Autodesk Inventor part; units mm, degrees
ref_plane "Work Plane1" through (28, 0, 0) normal (1, 0, 0) x (0, 1, 0)
ref_plane "XZ Plane" through (0, 0, 0) normal (0, 1, 0) x (-1, 0, 0)
ref_plane "XY Plane" through (0, 0, 0) normal (0, 0, 1) x (1, 0, 0)
sketch "Sketch1" plane through (0, 0, 0) normal (1, 0, 0) x (0, 1, 0)
  line L0 (-21.15, 21.15) -> (21.15, 21.15)
  line L1 (21.15, 21.15) -> (21.15, -21.15)
  line L2 (21.15, -21.15) -> (-21.15, -21.15)
  line L3 (-21.15, -21.15) -> (-21.15, 21.15)
  point P0 (0, 0)
  point P1 (0, 21.15)
  point P2 (21.15, 0)
  dimension "d0" = 42.3
  dimension "d1" = 42.3
extrude "Extrusion1" add sketch "Sketch1" along normal mid plane 56
ref_plane "Work Plane1" through (28, 0, 0) normal (1, 0, 0) x (0, 1, 0)
sketch "Sketch2" plane through (28, 0, 0) normal (1, 0, 0) x (0, 1, 0)
  circle A0 centre (0, 0) radius 11
  circle A1 centre (0, 0) radius 2.5
  circle A2 centre (15.5, 15.5) radius 2.55
  line L0 (21.15, -21.15) -> (21.15, 21.15) construction
  line L1 (21.15, 0) -> (0, 0) construction
  line L2 (0, 0) -> (0, 21.15) construction
  line L3 (21.15, 21.15) -> (-21.15, 21.15) construction
  circle A3 centre (15.5, -15.5) radius 2.55
  circle A4 centre (-15.5, 15.5) radius 2.55
  circle A5 centre (-15.5, -15.5) radius 2.55
  line L4 (1, 2.2913) -> (1, -2.2913)
  dimension "d5" = 22
  dimension "d6" = 5
  dimension "d15" = 5.1
  dimension "d16" = 31
  dimension "d17" = 31
  dimension "d20" = 1
extrude "Extrusion2" add sketch "Sketch2" along normal blind 2 contours A0
fillet "Fillet1" radius 2 1 edges at (0, 21.15, 21.15)
pattern_circular "Circular Pattern1" count 4 over 360 about axis through (28, 0, 0) along (1, 0, 0) of "Fillet1"
extrude "Extrusion4" cut sketch "Sketch2" against normal through all contours A2 | A3 | A4 | A5
sketch "Sketch3" plane through (0, 0, 0) normal (1, 0, 0) x (0, 1, 0)
  circle A0 centre (-15.5, 15.5) radius 2.55 construction
  circle A1 centre (15.5, 15.5) radius 2.55 construction
  circle A2 centre (-15.5, -15.5) radius 2.55 construction
  circle A3 centre (15.5, -15.5) radius 2.55 construction
  arc A4 (19.15, -21.15) -> (21.15, -19.15) centre (19.15, -19.15) ccw construction
  line L0 (21.15, -19.15) -> (21.15, 19.15) construction
  arc A5 (21.15, 19.15) -> (19.15, 21.15) centre (19.15, 19.15) ccw construction
  line L1 (19.15, 21.15) -> (-19.15, 21.15) construction
  arc A6 (-19.15, 21.15) -> (-21.15, 19.15) centre (-19.15, 19.15) ccw construction
  line L2 (-21.15, 19.15) -> (-21.15, -19.15) construction
  arc A7 (-21.15, -19.15) -> (-19.15, -21.15) centre (-19.15, -19.15) ccw construction
  line L3 (-19.15, -21.15) -> (19.15, -21.15) construction
  circle A8 centre (0, 0) radius 11 construction
  circle A9 centre (15.5, 15.5) radius 5.65 construction
  line L4 (-19.15, 21.15) -> (19.15, 21.15) construction
  line L5 (0, 21.15) -> (0, 0) construction
  line L6 (0, 0) -> (21.15, 0) construction
  line L7 (9.85, 15.5) -> (9.85, 21.15)
  line L8 (9.85, 21.15) -> (21.15, 21.15)
  line L9 (21.15, 21.15) -> (21.15, 9.85)
  line L10 (15.5, 9.85) -> (21.15, 9.85)
  arc A10 (9.85, 15.5) -> (15.5, 9.85) centre (15.5, 15.5) ccw
  circle A11 centre (15.5, -15.5) radius 2.55 construction
  arc A12 (19.15, -21.15) -> (21.15, -19.15) centre (19.15, -19.15) ccw construction
  circle A13 centre (0, 0) radius 11 construction
  circle A14 centre (15.5, -15.5) radius 5.65 construction
  line L11 (-19.15, -21.15) -> (19.15, -21.15) construction
  line L12 (9.85, -15.5) -> (9.85, -21.15)
  line L13 (9.85, -21.15) -> (21.15, -21.15)
  line L14 (21.15, -21.15) -> (21.15, -9.85)
  line L15 (15.5, -9.85) -> (21.15, -9.85)
  arc A15 (15.5, -9.85) -> (9.85, -15.5) centre (15.5, -15.5) ccw
  circle A16 centre (-15.5, 15.5) radius 2.55 construction
  circle A17 centre (-15.5, -15.5) radius 2.55 construction
  arc A18 (-21.15, -19.15) -> (-19.15, -21.15) centre (-19.15, -19.15) ccw construction
  arc A19 (-19.15, 21.15) -> (-21.15, 19.15) centre (-19.15, 19.15) ccw construction
  line L16 (19.15, -21.15) -> (-19.15, -21.15) construction
  circle A20 centre (-15.5, 15.5) radius 5.65 construction
  line L17 (-9.85, 15.5) -> (-9.85, 21.15)
  line L18 (-9.85, 21.15) -> (-21.15, 21.15)
  line L19 (-21.15, 21.15) -> (-21.15, 9.85)
  line L20 (-15.5, 9.85) -> (-21.15, 9.85)
  arc A21 (-15.5, 9.85) -> (-9.85, 15.5) centre (-15.5, 15.5) ccw
  circle A22 centre (-15.5, -15.5) radius 2.55 construction
  circle A23 centre (0, 0) radius 11 construction
  line L21 (-15.5, -9.85) -> (-21.15, -9.85)
  arc A24 (-9.85, -15.5) -> (-15.5, -9.85) centre (-15.5, -15.5) ccw
  line L22 (-9.85, -15.5) -> (-9.85, -21.15)
  line L23 (-21.15, -21.15) -> (-21.15, -9.85)
  line L24 (-9.85, -21.15) -> (-21.15, -21.15)
  arc A25 (-21.15, -19.15) -> (-19.15, -21.15) centre (-19.15, -19.15) ccw construction
  circle A26 centre (-15.5, -15.5) radius 5.65 construction
  point P0 (-21.15, 0)
  dimension "d25" = 11.3
extrude "Extrusion6" cut sketch "Sketch3" along normal mid plane 40
properties part number "stepper"
Source: CAD feature listing. Evaluate the final solid. Frame: model axes, mm. A direction names the side the tool comes from. Coordinates: 2 decimals unless noted, no trailing zeros. Loops run counter-clockwise (first coordinate to the right, second up) from the corner with the lowest first, then second, coordinate; pieces in that order, holes last. Notation, with made-up numbers: (85.25, 72.25) -> (113.25, 72.25) arc R23 cw to (113.25, 93.25) -> close; hole circle Ø6 at (80, 55). An arc over 180 degrees is marked (long way). Answer in a Markdown table with one row per item. Add a question column.
Q1. Section A-A on z = 0. Return the cut outline in (x, y), and give its area (3 significant figures).
Q2. Section C-C on x = 7. Return the cut outline in (y, z), and give its area (3 significant figures).
Q3. Ray query, line 1 along Z through (x, y) = (22.75, 15.5); line 2 along Z through (x, y) = (29.05, 0); line 3 along Y through (x, z) = (-23, 15). Return the intervals inside material, ascending.
Q4. Section D-D on y = 6.5. Return the cut outline in (x, z), and give its area (3 significant figures).
Q5. Reachability of faces 1 (the face through (28, -10, -9)), 2 (the face through (-0.28, -11.46, 11.55)), 3 (the face through (20, 17, 18)), 4 (the face through (0, 18, -9.85)) from +Z, -Z, +X, -X, +Y, -Y: full face, straight path, thin tool, end or side. Return the list, or none.
Q6. Contact query for flat-ended pins moving along their axis: pin 1 Ø3.5 at (y, z) = (-16.5, -15) entering from +X; pin 2 Ø3 at (y, z) = (-15.5, 15.5) entering from -X; pin 3 Ø4.5 at (x, y) = (8, 18.5) entering from -Z; pin 4 Ø1.5 at (x, y) = (-9, -16) entering from +Z. Output: stop coordinate, or through.
Q7. Pull-direction query (Z, two-part tool) for faces 5 (the face through (28, 0, 0)), 6 (the face through (-23.94, -20.55, 20.58)), 7 (the face through (-23.94, -20.58, -20.55)), 8 (the face through (-23.944, -17.524, 13.948)); classes: pulls with the +Z half, pulls with the -Z half, needs draft (parallel to the pull), parting line crosses it, or undercut.
Computed values:
| question | item | result |
|---|---|---|
| 1 | outline | (-28, -21.15) -> (28, -21.15) -> (28, -11) -> (30, -11) -> (30, -2.5) -> (28, -2.5) -> (28, 2.5) -> (30, 2.5) -> (30, 11) -> (28, 11) -> (28, 21.15) -> (-28, 21.15) -> close |
| 1 | area | 2,400 mm^2 |
| 2 | outline | (-21.15, -9.85) -> (-15.5, -9.85) arc R5.65 cw to (-9.85, -15.5) -> (-9.85, -21.15) -> (9.85, -21.15) -> (9.85, -15.5) arc R5.65 cw to (15.5, -9.85) -> (21.15, -9.85) -> (21.15, 9.85) -> (15.5, 9.85) arc R5.65 cw to (9.85, 15.5) -> (9.85, 21.15) -> (-9.85, 21.15) -> (-9.85, 15.5) arc R5.65 cw to (-15.5, 9.85) -> (-21.15, 9.85) -> close |
| 2 | area | 1,310 mm^2 |
| 3 | line 1 | z = -21.15 to -18.05, -12.95 to 12.95, 18.05 to 21.15 |
| 3 | line 2 | z = -11 to -2.5, 2.5 to 11 |
| 3 | line 3 | y = -21.15 to -18, -13 to 13, 18 to 21.15 |
| 4 | outline | (-28, -21.15) -> (28, -21.15) -> (28, -8.87) -> (30, -8.87) -> (30, 8.87) -> (28, 8.87) -> (28, 21.15) -> (-28, 21.15) -> close |
| 4 | area | 2,400 mm^2 |
| 5 | face 1 | +X |
| 5 | face 2 | +Z, -Y |
| 5 | face 3 | +Z, +Y |
| 5 | face 4 | -Z, +Y |
| 6 | pin 1 | stops at x = 28 |
| 6 | pin 2 | passes through |
| 6 | pin 3 | stops at z = -9.85 |
| 6 | pin 4 | stops at z = 9.86 |
| 7 | face 5 | undercut |
| 7 | face 6 | pulls with the +Z half |
| 7 | face 7 | pulls with the -Z half |
| 7 | face 8 | undercut |
